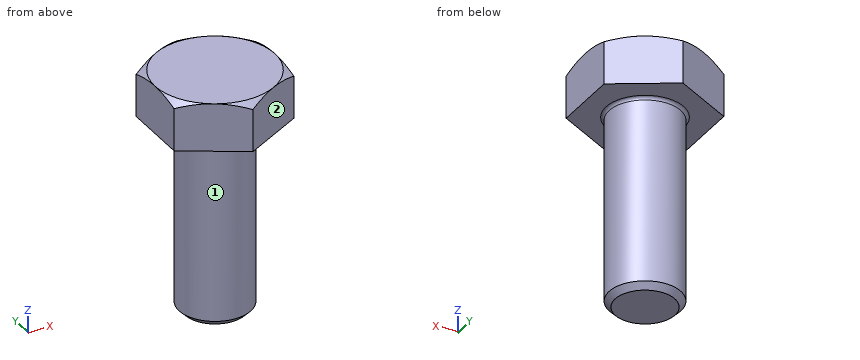
Autodesk Inventor part; units mm, degrees
ref_plane "WorkPlane1" through (0, 0, 0) normal (0, 0, 1) x (1, 0, 0)
ref_plane "MSC_PF1" through (0, 0, 0) normal (1, 0, 0) x (0, 1, 0)
ref_plane "MSC_PT1" through (0, 0, 0) normal (0, 0, -1) x (-1, 0, 0)
ref_plane "WorkPlane1" through (0, 0, 0) normal (0, 0, 1) x (1, 0, 0)
sketch "Sketch1" plane through (0, 0, 0) normal (0, 0, 1) x (1, 0, 0)
  point P0 (0, 0)
sketch "Sketch2" plane through (0, 0, 0) normal (0, 0, 1) x (1, 0, 0)
  line L0 (-5, 2.8868) -> (-5, -2.8868)
  line L1 (0, 5.7734) -> (-5, 2.8868)
  line L2 (5, 2.8868) -> (0, 5.7734)
  line L3 (5, -2.8868) -> (5, 2.8868)
  line L4 (0, -5.7734) -> (5, -2.8868)
  line L5 (-5, -2.8868) -> (0, -5.7734)
  circle A0 centre (0, 0) radius 5 construction
  dimension "d1" = 10
  dimension "d29" = 0
  dimension "d30" = 0
extrude "Extrusion1" add sketch "Sketch2" along normal blind 4
sketch "Sketch3" plane through (0, 0, 0) normal (1, 0, 0) x (0, 1, 0)
  line L0 (5, 4) -> (5.8734, 4)
  line L1 (5.8734, 3.4957) -> (5, 4)
  line L2 (5.8734, 4) -> (5.8734, 3.4957)
  line L3 (0, -0.8) -> (0, 4.8)
  line L4 (5.7734, 0) -> (5.7734, 4)
  dimension "d25" = 0.1
  dimension "d26" = 0
  dimension "d27" = 60
  dimension "d28" = 5
revolve "Revolution1" cut sketch "Sketch3" angle 360 about axis through (0, 0, -10) along (0, 0, 1)
sketch "Sketch4" plane through (0, 0, 0) normal (1, 0, 0) x (0, 1, 0)
  line L0 (0, -16) -> (0, 0)
  line L1 (-3, -16) -> (0, -16)
  line L2 (-3, 0) -> (-3, -16)
  line L3 (0, 0) -> (-3, 0)
  line L4 (0, -16) -> (0, 0)
  line L5 (-3.6, 0) -> (0.6, 0)
  line L6 (0, -19.2) -> (0, 3.2)
  dimension "d18" = 3
  dimension "d20" = 16
  dimension "d33" = 0
  dimension "d34" = 0
revolve "Revolution2" add sketch "Sketch4" angle 360 about axis through (0, 0, -16) along (0, 0, -1)
chamfer "Chamfer1" distance 0.5 angle 45 1 edges at (0, 3, -16)
fillet "Fillet1" radius 0.25 1 edges at (0, 3, 0)
thread "Thread1"
ref_plane "MSC_PF1" through (0, 0, 0) normal (1, 0, 0) x (0, 1, 0)
ref_plane "MSC_PT1" through (0, 0, 0) normal (0, 0, -1) x (-1, 0, 0)
equation "\"d22\" = 0.5 * PTC"
equation "\"d23\" = 0.5 * PTC"
equation "\"d24\" = r"
equation "\"d1\" = ParS"
equation "\"d6\" = ParK"
equation "\"b\" = NLG - 2 * PTC"
equation "\"d28\" = 0.5 * ParS"
equation "\"d18\" = 0.5 * NND"
equation "\"d20\" = NLG"
equation "\"NND\" = 6"
equation "\"NLG\" = 16"
equation "\"PTC\" = 1"
equation "\"ParK\" = 4"
equation "\"ParS\" = 10"
equation "\"msp_es\" = 0.577367 * ParS"
equation "\"r\" = 0.25"
equation "\"THREADDIA\" = NND"
properties part number "ISO 4018 - M6 x 16" material "Steel"
Geometry: final body of the model. Coordinates: model frame, mm. Face numbers are marked on the shaded views. A direction names the side the tool comes from. Give positions to 0.01 mm unless a question says otherwise; leave off trailing zeros. Write each loop counter-clockwise with the first axis right and the second up, starting at its lowest first coordinate (ties: lowest second). Pieces come first, ordered by that corner, then holes.
(1) Ray query, line 1 (Z direction, x = -4.5, y = -1.25); line 2 (X direction, y = -2.5, z = -11.5); line 3 (Y direction, x = 0.5, z = -0.5). Return the intervals inside material, ascending.
(2) First-contact query: P1, Ø4, axis at y = -2.5, z = -13.5, coming from the -X side; P2, Ø4, axis at x = 3, y = -4.5, coming from the +Z side; P3, Ø2, axis at y = 3, z = -9.5, coming from the +X side; P4, Ø1.5, axis at x = -2, z = 0, coming from the -Y side. Flat tips, straight axial feed; report the tip coordinate or a pass-through.
(3) Access query for the marked faces 1 and 2. Directions: +Z, -Z, +X, -X, +Y, -Y. A direction counts if a zero-diameter tool reaches every point of the face in a straight line with its end or side. Return the directions, or none.
(4) Cut plane A-A, the plane z = -8.5. Return loops of the section in (x, y).
Values follow:
1. line 1: z = 0 to 4
1. line 2: x = -1.66 to 1.66
1. line 3: y = -2.96 to 2.96
2. P1: stops at x = -2.96
2. P2: stops at z = 4
2. P3: stops at x = 2.24
2. P4: stops at y = -5.05
3. face 1: -Z
3. face 2: +Z, -Z, +X, -Y
4. outline: circle Ø6 at (0, 0)
